```python
from build123d import *

# Parameters (mm, degrees)
SKETCH1_W               = 70
SKETCH1_H               = 70
BOSS_EXTRUDE2_DEPTH     = 7
CUT_EXTRUDE1_DEPTH      = 5
SKETCH9_W               = 70
SKETCH9_H               = 70
BOSS_EXTRUDE3_DEPTH     = 5
CUT_EXTRUDE11_DEPTH     = 100.242128151
SKETCH21_R              = 3
CUT_EXTRUDE12_DEPTH     = 2
CHAMFER3_SIZE           = 1
CUT_EXTRUDE13_START     = -2
SKETCH22_W              = 70
SKETCH22_H              = 70
CUT_EXTRUDE13_DEPTH     = 2
SKETCH27_R              = 3
CUT_EXTRUDE27_DEPTH     = 2
SKETCH28_R              = 3
CUT_EXTRUDE28_DEPTH     = 2
MIRROR8_COPY_1_SKETCH_R = 3
MIRROR8_COPY_1_DEPTH    = 2
MIRROR8_COPY_2_SKETCH_R = 3
MIRROR8_COPY_2_DEPTH    = 2


with BuildPart() as part:
    # Sketch1 → Boss-Extrude2 (new body)
    with BuildSketch(Plane(origin=(0, 0, 0), x_dir=(1, 0, 0), z_dir=(0, 1, 0))):
        with Locations((35, 35)):
            Rectangle(SKETCH1_W, SKETCH1_H)
    extrude(amount=BOSS_EXTRUDE2_DEPTH)

    # Sketch3 → Cut-Extrude1 (cut)
    with BuildSketch(Plane(origin=(0, 7, 0), x_dir=(1, 0, 0), z_dir=(0, 1, 0))):
        with BuildLine():
            Line((2.5, 57.5), (2.5, 12.5))
            ThreePointArc((2.5, 12.5), (5.428932188, 5.428932188), (12.5, 2.5))
            Line((12.5, 2.5), (57.5, 2.5))
            ThreePointArc((57.5, 2.5), (64.571067812, 5.428932188), (67.5, 12.5))
            Line((67.5, 12.5), (67.5, 57.5))
            ThreePointArc((67.5, 57.5), (64.571067812, 64.571067812), (57.5, 67.5))
            Line((57.5, 67.5), (12.5, 67.5))
            ThreePointArc((12.5, 67.5), (5.428932188, 64.571067812), (2.5, 57.5))
        make_face()
    extrude(amount=-CUT_EXTRUDE1_DEPTH, mode=Mode.SUBTRACT)

    # Sketch9 → Boss-Extrude3 (add)
    with BuildSketch(Plane.XZ):
        with Locations((35, -35)):
            Rectangle(SKETCH9_W, SKETCH9_H)
    extrude(amount=BOSS_EXTRUDE3_DEPTH)

    # Sketch20 → Cut-Extrude11 (cut, through all)
    with BuildSketch(Plane(origin=(0, 2, 0), x_dir=(1, 0, 0), z_dir=(0, 1, 0))):
        with BuildLine():
            Line((13.745191882, 7.5), (56.254808118, 7.5))
            ThreePointArc((56.254808118, 7.5), (57.5, 12.5), (62.5, 13.745191882))
            Line((62.5, 13.745191882), (62.5, 56.254808118))
            ThreePointArc((62.5, 56.254808118), (57.5, 57.5), (56.254808118, 62.5))
            Line((56.254808118, 62.5), (13.745191882, 62.5))
            ThreePointArc((13.745191882, 62.5), (12.5, 57.5), (7.5, 56.254808118))
            Line((7.5, 56.254808118), (7.5, 13.745191882))
            ThreePointArc((7.5, 13.745191882), (12.5, 12.5), (13.745191882, 7.5))
        make_face()
    extrude(amount=-CUT_EXTRUDE11_DEPTH, mode=Mode.SUBTRACT)

    # Sketch21 → Cut-Extrude12 (cut)
    with BuildSketch(Plane(origin=(0, 2, 0), x_dir=(1, 0, 0), z_dir=(0, 1, 0))):
        with Locations(Location((8.964466094, 61.035533906, 0), (0, 0, 270))):
            Circle(SKETCH21_R)
        with Locations(Location((61.035533906, 61.035533906, 0), (0, 0, 270))):
            Circle(SKETCH21_R)
        with Locations(Location((61.035533906, 8.964466094, 0), (0, 0, 270))):
            Circle(SKETCH21_R)
        with Locations(Location((8.964466094, 8.964466094, 0), (0, 0, 270))):
            Circle(SKETCH21_R)
    extrude(amount=-CUT_EXTRUDE12_DEPTH, mode=Mode.SUBTRACT)

    # Chamfer3
    chamfer3_edges = [part.edges().sort_by_distance(p)[0] for p in [
        (5.428932188, 7, -5.428932188),
        (35, 7, -2.5),
        (64.571067812, 7, -5.428932188),
        (67.5, 7, -35),
        (64.571067812, 7, -64.571067812),
        (35, 7, -67.5),
        (5.428932188, 7, -64.571067812),
        (2.5, 7, -35),
        (12.5, 2, -12.5),
        (12.5, 2, -57.5),
        (57.5, 2, -57.5),
        (57.5, 2, -12.5),
        (35, 2, -7.5),
        (62.5, 2, -35),
        (35, 2, -62.5),
        (7.5, 2, -35),
    ]]
    chamfer(chamfer3_edges, length=CHAMFER3_SIZE)

    # Sketch22 → Cut-Extrude13 (cut)
    with BuildSketch(Plane.XZ.offset(5).offset(CUT_EXTRUDE13_START)):
        with Locations((35, -35)):
            Rectangle(SKETCH22_W, SKETCH22_H)
        with BuildLine():
            Line((7.5, -13.745191882), (7.5, -56.254808118))
            ThreePointArc((7.5, -56.254808118), (12.5, -57.5), (13.745191882, -62.5))
            Line((13.745191882, -62.5), (56.254808118, -62.5))
            ThreePointArc((56.254808118, -62.5), (57.5, -57.5), (62.5, -56.254808118))
            Line((62.5, -56.254808118), (62.5, -13.745191882))
            ThreePointArc((62.5, -13.745191882), (57.5, -12.5), (56.254808118, -7.5))
            Line((56.254808118, -7.5), (13.745191882, -7.5))
            ThreePointArc((13.745191882, -7.5), (12.5, -12.5), (7.5, -13.745191882))
        make_face(mode=Mode.SUBTRACT)
    extrude(amount=CUT_EXTRUDE13_DEPTH, mode=Mode.SUBTRACT)

    # Sketch27 → Cut-Extrude27 (cut)
    with BuildSketch(Plane.ZY):
        with Locations((-62.5, 2)):
            Circle(SKETCH27_R)
        with Locations((-7.5, 2)):
            Circle(SKETCH27_R)
    cut_extrude27 = extrude(amount=-CUT_EXTRUDE27_DEPTH, mode=Mode.SUBTRACT)

    # Sketch28 → Cut-Extrude28 (cut)
    with BuildSketch(Plane.XY):
        with Locations((7.5, 2)):
            Circle(SKETCH28_R)
        with Locations((62.5, 2)):
            Circle(SKETCH28_R)
    extrude(amount=-CUT_EXTRUDE28_DEPTH, mode=Mode.SUBTRACT)

    # Mirror2: part across plane


with BuildPart() as part_1:
    add(part.part)
    add(part.part.mirror(Plane(origin=(0, 7, -70), x_dir=(1, 0, 0), z_dir=(0, 0, 1))))

    # Mirror7: Cut-Extrude27 across plane
    add(cut_extrude27.mirror(Plane.ZY.offset(-35)), mode=Mode.SUBTRACT)

    # Mirror8 copy 1 sketch → Mirror8 copy 1 (cut)
    with BuildSketch(Plane(origin=(70, 0, -140), x_dir=(0, 0, -1), z_dir=(1, 0, 0))):
        with Locations((-62.5, 2)):
            Circle(MIRROR8_COPY_1_SKETCH_R)
        with Locations((-7.5, 2)):
            Circle(MIRROR8_COPY_1_SKETCH_R)
    extrude(amount=-MIRROR8_COPY_1_DEPTH, mode=Mode.SUBTRACT)

    # Mirror8 copy 2 sketch → Mirror8 copy 2 (cut)
    with BuildSketch(Plane(origin=(0, 0, -140), x_dir=(0, 0, -1), z_dir=(-1, 0, 0))):
        with Locations((-62.5, -2)):
            Circle(MIRROR8_COPY_2_SKETCH_R)
        with Locations((-7.5, -2)):
            Circle(MIRROR8_COPY_2_SKETCH_R)
    extrude(amount=-MIRROR8_COPY_2_DEPTH, mode=Mode.SUBTRACT)


solid = part_1.part
```
Geometry check sheet. Reference: the model listing, model coordinates, mm. A direction names the side the tool comes from. Coordinates: 2 decimals unless noted, no trailing zeros. Order: outer loops, then holes, each group sorted by start corner. A loop starts at its lowest first (then second) coordinate and runs counter-clockwise, first axis right, second up. Notation, with made-up numbers: (-39.75, -3.75) - (11.25, -3.75) arc R24 ccw to (11.25, 14.25) - close; hole circle Ø10 at (-23.5, 77). An arc over 180 degrees is marked (long way). Answer as a JSON object with one key per item and string values. Group by question number.
Item 1: Tool access check on faces 1 (the face through (61, 0, -79)), 2 (the face through (1, 0.2, -75.1)), 3 (the face through (69, 0.2, -64.9)), 4 (the face through (35, -1, -7.5)). Record the directions out of +Z, -Z, +X, -X, +Y, -Y that give a thin tool (end or side, any length) a straight path to the whole face; none if there is none.
Item 2: Scan lines: probe 1 along Z at (x, y) = (55, 4); probe 2 along Z at (x, y) = (28.5, 0); probe 3 along X at (y, z) = (2.5, -17). Record each from-to range of solid material in increasing order.
Item 3: Sectioned sample at A-A, the plane x = 18.5. Record the cut outline in (y, z), and give its area (3 significant figures).
Item 4: Sectioned sample at B-B, the plane z = -98. Record the cut outline in (x, y).
Item 5: Draft check along Z on faces 5 (the face through (62, 2, -2)), 6 (the face through (11.96, 1.84, -58.15)). Enter one of: +Z half, -Z half, draft (parallel to the pull), parting line (faces both ways), or undercut.
Item 6: Depth check by flat-ended pin: pin 1 Ø1.8 at (y, z) = (1.5, -7) entering from -X; pin 2 Ø7 at (x, z) = (8.96, -78.96) entering from +Y; pin 3 Ø1.8 at (y, z) = (2.5, -132.5) entering from +X; pin 4 Ø19.5 at (x, z) = (51, -31) entering from +Y. Enter the tip coordinate at first touch or a pass-through.
Resolved:
{
 "1": {"face 1": "+Y", "face 2": "-X", "face 3": "+X", "face 4": "+Y, -Y"},
 "2": {"probe 1": "-140 to -137.5, -72.5 to -67.5, -2.5 to 0", "probe 2": "-140 to -132.5, -77.5 to -62.5, -7.5 to 0", "probe 3": "0 to 2.5, 67.5 to 70"},
 "3": {"outline": "(-3, -140) - (7, -140) - (7, -138.5) - (6, -137.5) - (2, -137.5) - (2, -133.5) - (1, -132.5) - (-3, -132.5) - close; (-3, -77.5) - (1, -77.5) - (2, -76.5) - (2, -72.5) - (6, -72.5) - (7, -71.5) - (7, -68.5) - (6, -67.5) - (2, -67.5) - (2, -63.5) - (1, -62.5) - (-3, -62.5) - close; (-3, -7.5) - (1, -7.5) - (2, -6.5) - (2, -2.5) - (6, -2.5) - (7, -1.5) - (7, 0) - (-3, 0) - close", "area": "196 mm^2"},
 "4": {"outline": "(0, -3) - (7.5, -3) - (7.5, 1) - (6.5, 2) - (2.5, 2) - (2.5, 6) - (1.5, 7) - (0, 7) - close; (62.5, -3) - (70, -3) - (70, 7) - (68.5, 7) - (67.5, 6) - (67.5, 2) - (63.5, 2) - (62.5, 1) - close"},
 "5": {"face 5": "+Z half", "face 6": "undercut"},
 "6": {"pin 1": "x = 2", "pin 2": "y = 2", "pin 3": "x = 68", "pin 4": "through"}
}
